Read the model definition and answer for the solid it produces. Units are mm, in the model's axes. Face numbers are marked on the shaded views. Coordinates: 2 decimals unless noted, no trailing zeros. Order: outer loops, then holes, each group sorted by start corner. A loop starts at its lowest first (then second) coordinate and runs counter-clockwise, first axis right, second up. Notation, with made-up numbers: (23.5, -10) - (56.5, -10) arc R11 cw to (56.5, 1) - close; hole circle Ø9 at (-3.75, -38). An arc over 180 degrees is marked (long way). Write item = value, one per line.
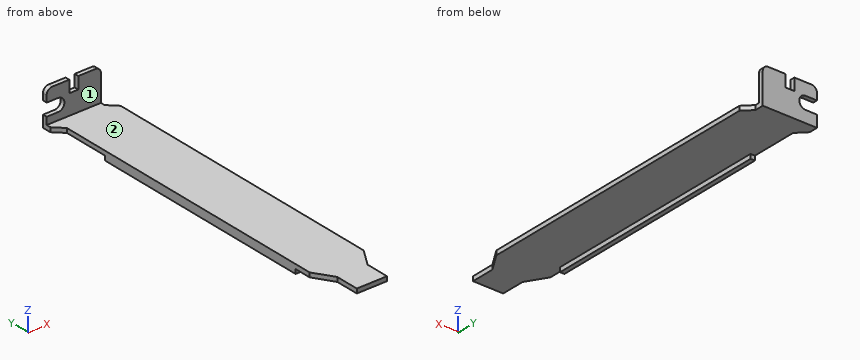
from build123d import *

# Parameters (mm, degrees)
F1_DEPTH = 1.5
F2_W     = 18.5
F2_H     = 1.5
F3_DEPTH = 10.9
F4_W     = 3.05
F4_H     = 4.1
F5_DEPTH = 25
F6_W     = 1.5
F6_H     = 78.4
F7_DEPTH = 1.5


with BuildPart() as f1:
    # F0 (on Top) → F1 (new body)
    with BuildSketch(Plane.XY):
        Polygon((-3.1, 103), (0, 99.9), (0, 0), (4.05, -6.5), (4.05, -14.5), (14.35, -14.5), (14.35, -6.5), (18.4, 0), (18.4, 100), (15.4, 103), (15.4, 106), (-3.1, 106), align=None)
    extrude(amount=F1_DEPTH)

    # F2 (on face) → F3 (join)
    with BuildSketch(Plane.XY.offset(1.5)):
        with Locations((6.15, 105.25)):
            Rectangle(F2_W, F2_H)
    extrude(amount=F3_DEPTH)

    # F4 (on face) → F5 (cut)
    with BuildSketch(Plane(origin=(0, 106, 0), x_dir=(-1, 0, 0), z_dir=(0, 1, 0))):
        with Locations((-6.15, 10.35)):
            Rectangle(F4_W, F4_H)
        with BuildLine():
            ThreePointArc((-15.4, 10.5), (-14.843503, 11.843503), (-13.5, 12.4))
            Line((-13.5, 12.4), (-15.4, 12.4))
            Line((-15.4, 12.4), (-15.4, 10.5))
        make_face()
        with BuildLine():
            Line((3.1, 12.4), (1.2, 12.4))
            ThreePointArc((1.2, 12.4), (2.543503, 11.843503), (3.1, 10.5))
            Line((3.1, 10.5), (3.1, 12.4))
        make_face()
        with BuildLine():
            Line((3.1, 8.26), (-0.8125, 8.26))
            ThreePointArc((-0.8125, 8.26), (-2.9425, 6.13), (-0.8125, 4))
            Line((-0.8125, 4), (3.1, 4))
            Line((3.1, 4), (3.1, 8.26))
        make_face()
    extrude(amount=-F5_DEPTH, mode=Mode.SUBTRACT)

    # F6 (on face) → F7 (join)
    with BuildSketch(Plane(origin=(0, 0, 0), x_dir=(1, 0, 0), z_dir=(0, 0, -1))):
        with Locations((0.75, -45)):
            Rectangle(F6_W, F6_H)
    extrude(amount=F7_DEPTH)


solid = f1.part
1) Straight lines are drawn through the part: line 1 along X through (y, z) = (25, 0.75); line 2 along Z through (x, y) = (8, 5.5); line 3 along Y through (x, z) = (12.5, 7.25). For each, find the intervals that lie inside material, in ascending order. Write a range as from..to.
Returned:
line_1 = 0..18.4
line_2 = 0..1.5
line_3 = 104.5..106
2) The part is cut by section D-D (y = 86). Determine the outline of the cut face in (x, z).
Returned:
outline = (0, 0) - (18.4, 0) - (18.4, 1.5) - (0, 1.5) - close
3) The part is cut by section C-C (z = 6.13). Determine the outline of the cut face in (x, y).
Returned:
outline = (2.94, 104.5) - (15.4, 104.5) - (15.4, 106) - (2.94, 106) - close
4) Determine the mould class of the marked faces 1 and 2 for opening direction Z: pulls with the +Z half, pulls with the -Z half, needs draft (parallel to the pull), parting line crosses it, or undercut.
Returned:
face_1 = needs draft
face_2 = pulls with the +Z half
5) Flat-ended cylindrical pins translate along their axes: pin 1 Ø1.6 at (x, z) = (1, -1) entering from +Y; pin 2 Ø6.5 at (x, y) = (11.5, 42.5) entering from -Z; pin 3 Ø8 at (x, z) = (12, 6.5) entering from -Y. Find the tip coordinate at first contact, or state that the pin passes through.
Returned:
pin_1 = 84.2
pin_2 = 0
pin_3 = 104.5
6) The part is cut by section A-A (y = 72). Determine the outline of the cut face in (x, z).
Returned:
outline = (0, -1.5) - (1.5, -1.5) - (1.5, 0) - (18.4, 0) - (18.4, 1.5) - (0, 1.5) - close
7) The part is cut by section B-B (x = 9.25). Determine the outline of the cut face in (y, z), and give its area (3 significant figures).
Returned:
outline = (-14.5, 0) - (106, 0) - (106, 12.4) - (104.5, 12.4) - (104.5, 1.5) - (-14.5, 1.5) - close
area = 197 mm^2
